Model file for the job. Use its own axes, mm. Face numbers are marked on the shaded views. A direction names the side the tool comes from. Round coordinates to 2 decimals unless told otherwise and drop trailing zeros. Order: outer loops, then holes, each group sorted by start corner. A loop starts at its lowest first (then second) coordinate and runs counter-clockwise, first axis right, second up. Notation, with made-up numbers: (-9, 37.5) -> (-4, 37.5) arc R24 ccw to (-4, 50.5) -> close; hole circle Ø3 at (54.25, 73). An arc over 180 degrees is marked (long way). Answer as CSV lines item,"result".
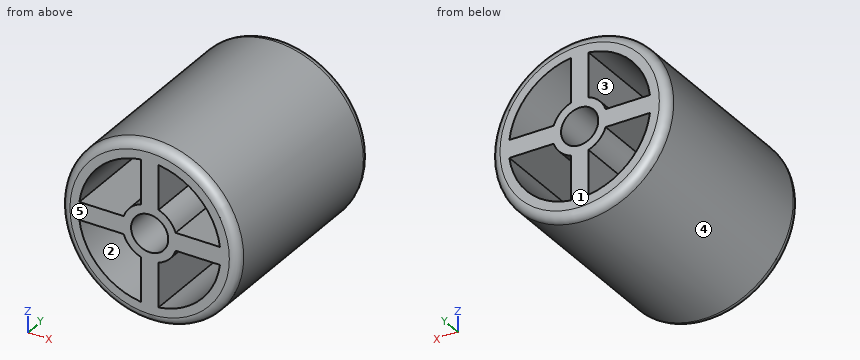
```python
from build123d import *

# Parameters (mm, degrees)
F0_R     = 5
F0_R_2   = 1.05
F1_DEPTH = 5.9
F2_R     = 0.5


with BuildPart() as f1:
    # F0 (on Front) → F1 (new body, symmetric)
    with BuildSketch(Plane.XZ):
        Circle(F0_R)
        with BuildLine():
            Line((-3.9686269666, -0.5), (-1.4671400751, -0.5))
            ThreePointArc((-1.4671400751, -0.5), (-1.0960155108, -1.0960155108), (-0.5, -1.4671400751))
            Line((-0.5, -1.4671400751), (-0.5, -3.9686269666))
            ThreePointArc((-0.5, -3.9686269666), (-2.8284271247, -2.8284271247), (-3.9686269666, -0.5))
        make_face(mode=Mode.SUBTRACT)
        with BuildLine():
            Line((1.4671400751, -0.5), (3.9686269666, -0.5))
            ThreePointArc((3.9686269666, -0.5), (2.8284271247, -2.8284271247), (0.5, -3.9686269666))
            Line((0.5, -3.9686269666), (0.5, -1.4671400751))
            ThreePointArc((0.5, -1.4671400751), (1.0960155108, -1.0960155108), (1.4671400751, -0.5))
        make_face(mode=Mode.SUBTRACT)
        with BuildLine():
            ThreePointArc((-3.9686269666, 0.5), (-2.8284271247, 2.8284271247), (-0.5, 3.9686269666))
            Line((-0.5, 3.9686269666), (-0.5, 1.4671400751))
            ThreePointArc((-0.5, 1.4671400751), (-1.0960155108, 1.0960155108), (-1.4671400751, 0.5))
            Line((-1.4671400751, 0.5), (-3.9686269666, 0.5))
        make_face(mode=Mode.SUBTRACT)
        Circle(F0_R_2, mode=Mode.SUBTRACT)
        with BuildLine():
            ThreePointArc((0.5, 3.9686269666), (2.8284271247, 2.8284271247), (3.9686269666, 0.5))
            Line((3.9686269666, 0.5), (1.4671400751, 0.5))
            ThreePointArc((1.4671400751, 0.5), (1.0960155108, 1.0960155108), (0.5, 1.4671400751))
            Line((0.5, 1.4671400751), (0.5, 3.9686269666))
        make_face(mode=Mode.SUBTRACT)
    extrude(amount=F1_DEPTH, both=True)

    # F2
    f2_edges = [f1.edges().sort_by_distance(p)[0] for p in [
        (-5, -5.9, 0),
        (-5, 5.9, 0),
    ]]
    fillet(f2_edges, radius=F2_R)


solid = f1.part
```
Q1. Saw through at D-D (z = 1.25). State how many separate pieces and enclosed holes the cut face has, plus the area to 3 significant figures.
Checks:
separate pieces,"3"
enclosed holes,"0"
area,"46.0 mm²"
Q2. Wall check: L1, parallel to Z at x = 0, y = 3.25; L2, parallel to Z at x = -3.5, y = 4; L3, parallel to X at y = -5, z = -3.25. Give the ranges that are in metal, low to high. Write a range as [from, to].
Checks:
L1,"[-5, -1.05], [1.05, 5]"
L2,"[-3.57, -1.94], [-0.5, 0.5], [1.94, 3.57]"
L3,"[-3.8, -2.33], [-0.5, 0.5], [2.33, 3.8]"
Q3. Saw through at B-B (z = 0). Write the cut outline in (x, y).
Checks:
outline,"(-5, -5.4) arc R0.5 ccw to (-4.5, -5.9) -> (-1.05, -5.9) -> (-1.05, 5.9) -> (-4.5, 5.9) arc R0.5 ccw to (-5, 5.4) -> close; (1.05, -5.9) -> (4.5, -5.9) arc R0.5 ccw to (5, -5.4) -> (5, 5.4) arc R0.5 ccw to (4.5, 5.9) -> (1.05, 5.9) -> close"
Q4. Saw through at A-A (x = 0). Write the cut outline in (y, z).
Checks:
outline,"(-5.9, -4.5) arc R0.5 ccw to (-5.4, -5) -> (5.4, -5) arc R0.5 ccw to (5.9, -4.5) -> (5.9, -1.05) -> (-5.9, -1.05) -> close; (-5.9, 1.05) -> (5.9, 1.05) -> (5.9, 4.5) arc R0.5 ccw to (5.4, 5) -> (-5.4, 5) arc R0.5 ccw to (-5.9, 4.5) -> close"
Q5. Saw through at C-C (y = -4.5). Write the cut outline in (x, z), plus the area to 3 significant figures.
Checks:
outline,"circle Ø10 at (0, 0); hole (-3.97, -0.5) arc R4 ccw to (-0.5, -3.97) -> (-0.5, -1.47) arc R1.55 cw to (-1.47, -0.5) -> close; hole (-3.97, 0.5) -> (-1.47, 0.5) arc R1.55 cw to (-0.5, 1.47) -> (-0.5, 3.97) arc R4 ccw to start; hole circle Ø2.1 at (0, 0); hole (0.5, -3.97) arc R4 ccw to (3.97, -0.5) -> (1.47, -0.5) arc R1.55 cw to (0.5, -1.47) -> close; hole (0.5, 1.47) arc R1.55 cw to (1.47, 0.5) -> (3.97, 0.5) arc R4 ccw to (0.5, 3.97) -> close"
area,"42.2 mm²"
Q6. Flat gauge pins, fed straight in: pin 1 (1 mm diameter, centred on x = -2, y = -3, fed in from -Z); pin 2 (1.3 mm diameter, centred on x = 3, y = 1.5, fed in from -Z); pin 3 (1.3 mm diameter, centred on y = 1, z = -2, fed in from +X). Where does each tip first touch, or does it go through?
Checks:
pin 1,"z = -4.77"
pin 2,"z = -4.41"
pin 3,"x = 4.81"
Q7. Mould opens along Z. For the marked faces 3, 4 and 5 say: +Z half, -Z half, draft (parallel to the pull), parting line (faces both ways), or undercut.
Checks:
face 3,"undercut"
face 4,"parting line"
face 5,"draft"
Q8. Tool access for the marked faces 1 and 2: list every direction of +Z, -Z, +X, -X, +Y, -Y with a clear straight run to the whole face (end or side of a thin tool).
Checks:
face 1,"+Z, -Z, +X, -X, +Y"
face 2,"+Y, -Y"
